Verification items for this drawing (mm, ordinates from the low corner). Round coordinates to 2 decimals unless told otherwise and drop trailing zeros. Write each loop counter-clockwise with the first axis right and the second up, starting at its lowest first coordinate (ties: lowest second). Pieces come first, ordered by that corner, then holes.
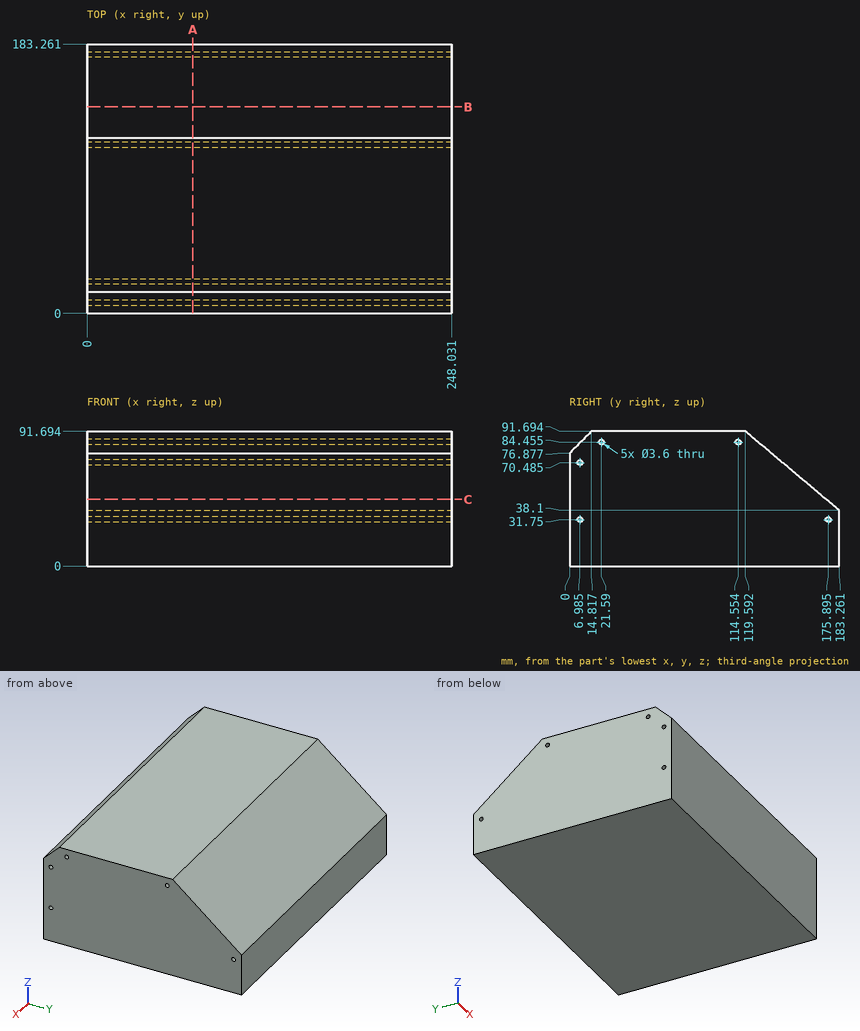
1. Section check B-B (y = 140.5). Record the cut outline in (x, z) (1 decimal), plus the area to 3 significant figures.
2. Section check C-C (z = 45.5). Record the cut outline in (x, y), plus the area to 3 significant figures.
3. Scan lines: line 1 along Z through (x, y) = (59.5, 126); line 2 along Y through (x, z) = (37.5, 31); line 3 along Z through (x, y) = (89, 21) (1 decimal). Record each from-to range of solid material in increasing order.
4. Depth check by flat-ended pin: pin 1 Ø8 at (x, z) = (198.5, 81.5) entering from -Y (1 decimal). Enter the tip coordinate at first touch or a pass-through.
5. Section check A-A (x = 72). State how many separate pieces and enclosed holes the cut face has, plus the area to 3 significant figures.
Results below:
1. outline: (0, 0) - (248, 0) - (248, 74.1) - (0, 74.1) - close
1. area: 18,400 mm2
2. outline: (0, 0) - (248.03, 0) - (248.03, 174.47) - (0, 174.47) - close
2. area: 43,300 mm2
3. line 1: z = 0 to 86.3
3. line 2: y = 0 to 5.35, 8.62 to 174.26, 177.53 to 183.26
3. line 3: z = 0 to 82.8, 86.2 to 91.7
4. pin 1: stops at y = 0.6
5. separate pieces: 1
5. enclosed holes: 5
5. area: 14,900 mm2
